```python
from build123d import *

# Parameters (mm, degrees)
BOSS_EXTRUDE1_DEPTH = 37.5


with BuildPart() as part:
    # Sketch1 → Boss-Extrude1 (new, symmetric)
    with BuildSketch(Plane(origin=(0, 0, 0), x_dir=(1, 0, 0), z_dir=(0, 1, 0))):
        with BuildLine():
            Line((-108, 24), (108, 24))
            ThreePointArc((108, 24), (115.424621202, 20.924621202), (118.5, 13.5))
            Line((118.5, 13.5), (118.5, -24))
            Line((118.5, -24), (-118.5, -24))
            Line((-118.5, -24), (-118.5, 13.5))
            ThreePointArc((-118.5, 13.5), (-115.424621202, 20.924621202), (-108, 24))
        make_face()
    extrude(amount=BOSS_EXTRUDE1_DEPTH, both=True)


solid = part.part
```
Can you work these out from the model? Positions are in its coordinate system, mm. Round coordinates to 2 decimals unless told otherwise and drop trailing zeros. Loops run counter-clockwise (first coordinate to the right, second up) from the corner with the lowest first, then second, coordinate; pieces in that order, holes last.
Item 1: Suppose I cut it at A-A, the plane z = -20. Write out the boundary of the cut face in (x, y), then the cut area to 3 significant figures.
Item 2: Will this pin go through, and if not, where does the flat tip stop? pin 1 Ø6 at (y, z) = (-23.5, -17.5) entering from +X.
Item 3: Please list where these lines run through material, in increasing order: L1, parallel to X at y = -17, z = -14; L2, parallel to X at y = 1, z = -19.5.
Reported:
1. outline: (-116.25, -37.5) - (116.25, -37.5) - (116.25, 37.5) - (-116.25, 37.5) - close
1. area: 17,400 mm2
2. pin 1: stops at x = 118.45
3. L1: x = -118.49 to 118.49
3. L2: x = -116.62 to 116.62
